Read the model definition and answer for the solid it produces. Units are mm, in the model's axes. A direction names the side the tool comes from. Coordinates: 2 decimals unless noted, no trailing zeros. Write each loop counter-clockwise with the first axis right and the second up, starting at its lowest first coordinate (ties: lowest second). Pieces come first, ordered by that corner, then holes. Notation, with made-up numbers: (10.25, 14.25) -> (55.25, 14.25) arc R12 cw to (55.25, 29.25) -> close; hole circle Ø4 at (-37.5, -4.75). An arc over 180 degrees is marked (long way). Answer in a Markdown table with one row per item. Add a question column.
Item 1: Given pin 1 Ø11.5 at (x, y) = (0, 96.5) entering from -Z; pin 2 Ø5 at (x, z) = (6.5, 15) entering from -Y; pin 3 Ø4 at (y, z) = (95.95, 15) entering from -X; pin 4 Ø10 at (x, z) = (-5.5, 4) entering from -Y, each flat-ended and moving along its own axis, determine where each tip first touches the part or whether it passes through.
Item 2: Section A-A on z = 10 is taken. Write down the section's boundary in (x, y).
Item 3: Which of the six approach directions +Z, -Z, +X, -X, +Y, -Y give full straight-line access (tool end or side, diameter ignored) to faces 5 (the face through (-5, 96, 10)), 6 (the face through (-0.74, 17.484, 9.965)), 7 (the face through (-7.33, 97.19, 15.16))?
Item 4: For a pull along X with two mould halves and no side action, classify faces 1 (the face through (0, 88.9, 7)), 2 (the face through (0, 48, 0)), 3 (the face through (0, 96, 7.5)), 4 (the face through (-5.61, -0.47, 4.2)) as +X half, -X half, draft (parallel to the pull), parting line (faces both ways), or undercut.
Item 5: Straight lines are drawn through the part: line 1 (Z direction, x = 6.75, y = 95.95); line 2 (X direction, y = 94, z = 9); line 3 (Y direction, x = -7.75, z = 5). For each, find the intervals that lie inside material, in ascending order. Write a range as from..to.
```python
from build123d import *

# Parameters (mm, degrees)
BOSS_EXTRUDE1_DEPTH             = 7.5
BOSS_EXTRUDE2_DEPTH             = 5
BOSS_EXTRUDE3_DEPTH             = 7.5
SKETCH4_R                       = 3
CUT_EXTRUDE1_DEPTH              = 106.399240984
CUT_EXTRUDE2_DEPTH              = 14.1
FILLET1_R                       = 1
M3X0_5_TAPPED_HOLE1_D           = 2.5
M3X0_5_TAPPED_HOLE1_DEPTH       = 18
M3X0_5_TAPPED_HOLE1_CSINK_D     = 5.6
M3X0_5_TAPPED_HOLE1_CSINK_ANGLE = 90
M3X0_5_TAPPED_HOLE1_TIP         = 0.751075774


with BuildPart() as part:
    # Sketch1 → Boss-Extrude1 (new body)
    with BuildSketch(Plane.XY):
        with BuildLine():
            Line((0, -10), (0, -5))
            ThreePointArc((0, -5), (-2.886751346, -4.082482905), (-4.714045208, -1.666666667))
            ThreePointArc((-4.714045208, -1.666666667), (-5.627692139, -0.458758548), (-7.071067812, 0))
            Line((-7.071067812, 0), (-7.5, 0))
            ThreePointArc((-7.5, 0), (-9.267766953, 0.732233047), (-10, 2.5))
            Line((-10, 2.5), (-10, 103))
            Line((-10, 103), (10, 103))
            Line((10, 103), (10, 0))
            ThreePointArc((10, 0), (7.071067812, -7.071067812), (0, -10))
        make_face()
    extrude(amount=BOSS_EXTRUDE1_DEPTH)

    # Sketch2 → Boss-Extrude2 (add)
    with BuildSketch(Plane.XY.offset(7.5)):
        with BuildLine():
            Line((-10, 103), (10, 103))
            Line((10, 103), (10, 14.361406616))
            ThreePointArc((10, 14.361406616), (0, 17.5), (-10, 14.361406616))
            Line((-10, 14.361406616), (-10, 103))
        make_face()
    extrude(amount=BOSS_EXTRUDE2_DEPTH)

    # Sketch3 → Boss-Extrude3 (add)
    with BuildSketch(Plane.XY.offset(12.5)):
        with BuildLine():
            Line((7.447916037, -0.882352941), (10, 20.659715081))
            Line((10, 20.659715081), (10, 103))
            Line((10, 103), (-10, 103))
            Line((-10, 103), (-10, 0))
            Line((-10, 0), (-7.5, 0))
            ThreePointArc((-7.5, 0), (-0.441944412, -7.486967686), (7.447916037, -0.882352941))
        make_face()
    extrude(amount=BOSS_EXTRUDE3_DEPTH)

    # Sketch4 → Cut-Extrude1 (cut, through all)
    with BuildSketch(Plane(origin=(0, 0, 0), x_dir=(-1, 0, 0), z_dir=(0, 0, -1))):
        Circle(SKETCH4_R)
    extrude(amount=-CUT_EXTRUDE1_DEPTH, mode=Mode.SUBTRACT)

    # Sketch5 → Cut-Extrude2 (cut)
    with BuildSketch(Plane(origin=(0, 103, 0), x_dir=(1, 0, 0), z_dir=(0, 1, 0))):
        with BuildLine():
            Line((-5.25, -17.5), (5.25, -17.5))
            ThreePointArc((5.25, -17.5), (5.957106781, -17.207106781), (6.25, -16.5))
            Line((6.25, -16.5), (6.25, -3.5))
            ThreePointArc((6.25, -3.5), (5.957106781, -2.792893219), (5.25, -2.5))
            Line((5.25, -2.5), (-5.25, -2.5))
            ThreePointArc((-5.25, -2.5), (-5.957106781, -2.792893219), (-6.25, -3.5))
            Line((-6.25, -3.5), (-6.25, -16.5))
            ThreePointArc((-6.25, -16.5), (-5.957106781, -17.207106781), (-5.25, -17.5))
        make_face()
        with BuildLine():
            Line((-4, -12.5), (4, -12.5))
            ThreePointArc((4, -12.5), (4.707106781, -12.207106781), (5, -11.5))
            Line((5, -11.5), (5, -8.5))
            ThreePointArc((5, -8.5), (4.707106781, -7.792893219), (4, -7.5))
            Line((4, -7.5), (-4, -7.5))
            ThreePointArc((-4, -7.5), (-4.707106781, -7.792893219), (-5, -8.5))
            Line((-5, -8.5), (-5, -11.5))
            ThreePointArc((-5, -11.5), (-4.707106781, -12.207106781), (-4, -12.5))
        make_face(mode=Mode.SUBTRACT)
    extrude(amount=-CUT_EXTRUDE2_DEPTH, mode=Mode.SUBTRACT)

    # Fillet1
    # the kernel refuses this fillet: 1 mm, written as the material it takes off along each edge
    with BuildSketch(Plane(origin=(10, 105.5, 0), x_dir=(-1, 0, 0), z_dir=(0, -1, 0))) as fillet1_piece_1:
        with BuildLine():
            CenterArc((FILLET1_R, -FILLET1_R), FILLET1_R, 90, 90)
            Line((0, -FILLET1_R), (0, 0))
            Line((0, 0), (FILLET1_R, 0))
        make_face()
    extrude(amount=105.5, mode=Mode.SUBTRACT)
    with BuildSketch(Plane(origin=(0, 0, 0), x_dir=(1, 0, 0), z_dir=(0, 1, 0))) as fillet1_piece_2:
        with BuildLine():
            CenterArc((10 - FILLET1_R, -FILLET1_R), FILLET1_R, 0, 90)
            Line((10 - FILLET1_R, 0), (10, 0))
            Line((10, 0), (10, -FILLET1_R))
        make_face()
    revolve(axis=Axis((0, 0, 0), (0, 0, -1)), revolution_arc=104.329698924, mode=Mode.SUBTRACT)
    with BuildSketch(Plane(origin=(0, 0, 0), x_dir=(0, -1, 0), z_dir=(1, 0, 0))) as fillet1_piece_3:
        with BuildLine():
            CenterArc((5 - FILLET1_R, -FILLET1_R), FILLET1_R, 0, 90)
            Line((5 - FILLET1_R, 0), (5, 0))
            Line((5, 0), (5, -FILLET1_R))
        make_face()
    revolve(axis=Axis((0, 0, 0), (0, 0, -1)), revolution_arc=70.528779366, mode=Mode.SUBTRACT)
    with BuildSketch(Plane(origin=(-7.071067812, -2.5, 0), x_dir=(0.9428090415820636, 0.3333333333333328, 0), z_dir=(0.3333333333333328, -0.9428090415820636, 0))) as fillet1_piece_4:
        with BuildLine():
            CenterArc((2.5 + FILLET1_R, FILLET1_R), FILLET1_R, 180, 90)
            Line((2.5, FILLET1_R), (2.5, 0))
            Line((2.5, 0), (2.5 + FILLET1_R, 0))
        make_face()
    revolve(axis=Axis((-7.071067812, -2.5, 0), (0, 0, 1)), revolution_arc=70.528779366, mode=Mode.SUBTRACT)
    with BuildSketch(Plane(origin=(0, -10, -2.782087795), x_dir=(0, 1, 0), z_dir=(0, 0, 1))) as fillet1_piece_5:
        with BuildLine():
            CenterArc((1.05572809, -1), FILLET1_R, 90, 96.379370208)
            ThreePointArc((0.0619201, -1.111111111), (0.015492025, -0.556417559), (0, 0))
            Line((0, 0), (1.05572809, 0))
        make_face()
    extrude(amount=13.06417559, mode=Mode.SUBTRACT)
    with BuildSketch(Plane(origin=(10, 14.361406616, 7.5), x_dir=(0, 1, 0), z_dir=(0, 0, 1))) as fillet1_piece_6:
        with BuildLine():
            CenterArc((1.801823259, 1), FILLET1_R, 150.89009106, 119.10990894)
            ThreePointArc((0.928135158, 1.486486486), (0.482686338, 0.731618028), (0, 0))
            Line((0, 0), (1.801823259, 0))
        make_face()
    extrude(amount=5, mode=Mode.SUBTRACT)
    with BuildSketch(Plane(origin=(-10, 0, 10), x_dir=(0, 1, 0), z_dir=(0, 0, 1))) as fillet1_piece_7:
        with BuildLine():
            CenterArc((FILLET1_R, -FILLET1_R), FILLET1_R, 90, 90)
            Line((0, -FILLET1_R), (0, 0))
            Line((0, 0), (FILLET1_R, 0))
        make_face()
    extrude(amount=12.5, mode=Mode.SUBTRACT)
    with BuildSketch(Plane(origin=(10, 8.159715081, 20), x_dir=(0, 0, -1), z_dir=(0, 1, 0))) as fillet1_piece_8:
        with BuildLine():
            CenterArc((FILLET1_R, FILLET1_R), FILLET1_R, 180, 90)
            Line((0, FILLET1_R), (0, 0))
            Line((0, 0), (FILLET1_R, 0))
        make_face()
    extrude(amount=97.340284919, mode=Mode.SUBTRACT)
    with BuildSketch(Plane(origin=(-10, 105.5, 20), x_dir=(0, 0, -1), z_dir=(0, -1, 0))) as fillet1_piece_9:
        with BuildLine():
            CenterArc((FILLET1_R, FILLET1_R), FILLET1_R, 180, 90)
            Line((0, FILLET1_R), (0, 0))
            Line((0, 0), (FILLET1_R, 0))
        make_face()
    extrude(amount=108, mode=Mode.SUBTRACT)
    with BuildSketch(Plane(origin=(-7.071067812, 0, 0), x_dir=(0, 1, 0), z_dir=(-1, 0, 0))) as fillet1_piece_10:
        with BuildLine():
            CenterArc((FILLET1_R, -FILLET1_R), FILLET1_R, 90, 90)
            Line((0, -FILLET1_R), (0, 0))
            Line((0, 0), (FILLET1_R, 0))
        make_face()
    extrude(amount=0.428932188, mode=Mode.SUBTRACT)
    with BuildSketch(Plane(origin=(-7.5, 2.5, 0), x_dir=(0, -1, 0), z_dir=(1, 0, 0))) as fillet1_piece_11:
        with BuildLine():
            CenterArc((2.5 - FILLET1_R, -FILLET1_R), FILLET1_R, 0, 90)
            Line((2.5, -FILLET1_R), (2.5, 0))
            Line((2.5, 0), (2.5 - FILLET1_R, 0))
        make_face()
    revolve(axis=Axis((-7.5, 2.5, 0), (0, 0, -1)), revolution_arc=90, mode=Mode.SUBTRACT)
    with BuildSketch(Plane(origin=(-10, 2.5, 0), x_dir=(1, 0, 0), z_dir=(0, 1, 0))) as fillet1_piece_12:
        with BuildLine():
            CenterArc((FILLET1_R, -FILLET1_R), FILLET1_R, 90, 90)
            Line((0, -FILLET1_R), (0, 0))
            Line((0, 0), (FILLET1_R, 0))
        make_face()
    extrude(amount=103, mode=Mode.SUBTRACT)

    # M3x0.5 Tapped Hole1
    with Locations(Plane.ZY.offset(10)):
        with Locations((15, 95.95), (5, 95.95)):
            CounterSinkHole(M3X0_5_TAPPED_HOLE1_D / 2, M3X0_5_TAPPED_HOLE1_CSINK_D / 2, depth=M3X0_5_TAPPED_HOLE1_DEPTH, counter_sink_angle=M3X0_5_TAPPED_HOLE1_CSINK_ANGLE)
            with Locations((0, 0, -(M3X0_5_TAPPED_HOLE1_DEPTH + M3X0_5_TAPPED_HOLE1_TIP / 2))):  # 118° drill point
                Cone(0, M3X0_5_TAPPED_HOLE1_D / 2, M3X0_5_TAPPED_HOLE1_TIP, mode=Mode.SUBTRACT)


solid = part.part
```
Results below:
| question | item | result |
|---|---|---|
| 1 | pin 1 | stops at z = 0 |
| 1 | pin 2 | stops at y = -6.34 |
| 1 | pin 3 | stops at x = -9.2 |
| 1 | pin 4 | stops at y = -4.97 |
| 2 | outline | (-10, 14.36) arc R17.5 cw to (8.51, 15.29) arc R1 ccw to (10, 16.16) -> (10, 103) -> (6.25, 103) -> (6.25, 88.9) -> (5, 88.9) -> (5, 103) -> (-5, 103) -> (-5, 88.9) -> (-6.25, 88.9) -> (-6.25, 103) -> (-10, 103) -> close |
| 3 | face 5 | +Y |
| 3 | face 6 | -Y |
| 3 | face 7 | -X |
| 4 | face 1 | undercut |
| 4 | face 2 | draft |
| 4 | face 3 | undercut |
| 4 | face 4 | -X half |
| 5 | line 1 | z = 0..3.75, 6.25..13.75, 16.25..20 |
| 5 | line 2 | x = -10..-6.25, -5..5, 6.25..10 |
| 5 | line 3 | y = 0.01..94.7, 97.2..103 |
